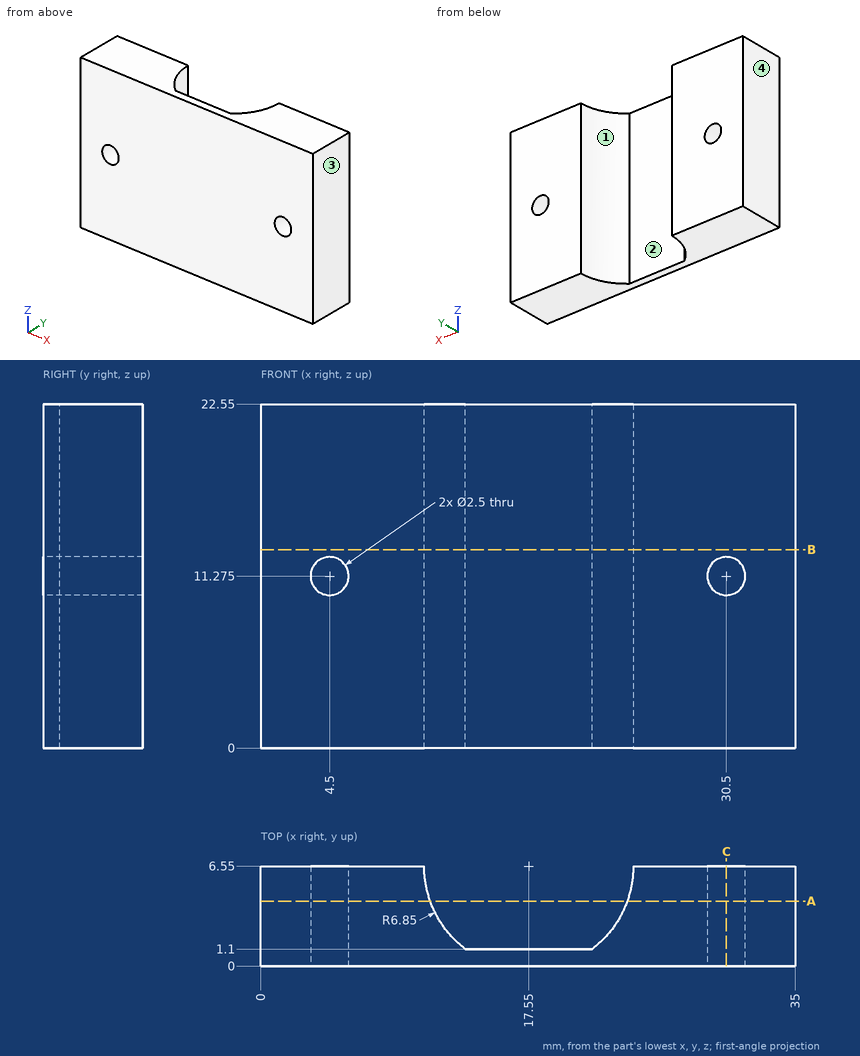
Print and shaded views of the part. All mm, measured from the part's lowest x, y and z. Coordinates: 2 decimals unless noted, no trailing zeros. Loops run counter-clockwise (first coordinate to the right, second up) from the corner with the lowest first, then second, coordinate; pieces in that order, holes last. Notation, with made-up numbers: (-24, -23.5) - (-3, -23.5) arc R30 ccw to (-3, 4.5) - close; hole circle Ø10 at (73.5, 34.25). An arc over 180 degrees is marked (long way). Write item = value, one per line. Start each with the question number.
Item 1: Wall check: L1, parallel to X at y = 2, z = 10.5; L2, parallel to X at y = 4.75, z = 11; L3, parallel to X at y = 6.25, z = 14.5. Give the ranges that are in metal, low to high. Write a range as from..to.
Item 2: Cut at C-C, the plane x = 30.5. Give the cut face in (y, z) (3 decimals).
Item 3: Mould opens along X. For the marked faces 1, 2, 3 and 4 say: released by +X, released by -X, zero draft, split by the parting line, or undercut.
Item 4: Cut at B-B, the plane z = 13. Give the cut face in (x, y), and give its area (3 significant figures).
Item 5: Flat gauge pins, fed straight in: pin 1 Ø1.5 at (y, z) = (2.5, 3) entering from -X; pin 2 Ø2 at (x, z) = (30.5, 11.275) entering from -Y; pin 3 Ø6.5 at (x, z) = (18, 8) entering from +Y. Where does each tip first touch, or does it go through?
Item 6: Cut at A-A, the plane y = 4.25. Give the cut face in (x, z) (3 decimals), and give its area (3 significant figures).
The answers:
q1.L1 = 0..3.52, 5.48..12.43, 22.67..29.52, 31.48..35
q1.L2 = 0..3.28, 5.72..10.94, 24.16..29.28, 31.72..35
q1.L3 = 0..10.71, 24.39..35
q2.outline = (0, 0) - (6.55, 0) - (6.55, 10.025) - (0, 10.025) - close; (0, 12.525) - (6.55, 12.525) - (6.55, 22.55) - (0, 22.55) - close
q3.face_1 = undercut
q3.face_2 = undercut
q3.face_3 = released by +X
q3.face_4 = released by -X
q4.outline = (0, 0) - (35, 0) - (35, 6.55) - (24.4, 6.55) arc R6.85 cw to (21.7, 1.1) - (13.4, 1.1) arc R6.85 cw to (10.7, 6.55) - (0, 6.55) - close
q4.area = 163 mm2
q5.pin_1 = 0
q5.pin_2 = through
q5.pin_3 = 1.1
q6.outline = (0, 0) - (11.098, 0) - (11.098, 22.55) - (0, 22.55) - close; (24.002, 0) - (35, 0) - (35, 22.55) - (24.002, 22.55) - close; hole circle Ø2.5 at (4.5, 11.275); hole circle Ø2.5 at (30.5, 11.275)
q6.area = 488 mm2
